The model under review builds one solid part; all positions refer to its coordinate system, in mm. A direction names the side the tool comes from. Round coordinates to 2 decimals unless told otherwise and drop trailing zeros. Order: outer loops, then holes, each group sorted by start corner. A loop starts at its lowest first (then second) coordinate and runs counter-clockwise, first axis right, second up. Notation, with made-up numbers: M 2.25,68.5 L 43.25,68.5 A25 cw 43.25,98.5 Z; hole C 44.5,76.25 d1. An arc over 180 degrees is marked long. Answer as a JSON object with one key per item and string values. Group by question number.
1) For faces 3 (the cylindrical face through (219.16, -261.17, -174.237)), 4 (the flat face through (70, 253, -40)), 5 (the flat face through (281, -266, -164)), 6 (the flat face through (315, 0, 0)), 7 (the flat face through (-4, -250, -1)), list the 3-axis set-ups (+Z, -Z, +X, -X, +Y, -Y) from which the entire face can be reached by the end or side of a thin tool; tool diameter is ignored.
2) Consider section C-C, the plane y = 72.5. Write out the cut boundary in (x, z), then the cut area to 3 significant figures.
3) Consider section A-A, the plane z = -40. Write out the cut boundary in (x, y).
4) Consider section B-B, the plane x = 135.5. Write out the cut boundary in (y, z).
5) To check wall thickness, follow line 1 (X direction, y = 255.5, z = 40); line 2 (Y direction, x = -277, z = -76.5); line 3 (X direction, y = 225, z = -119). State the ranges of each line that lie inside material, in increasing order.
6) Consider section D-D, the plane x = -7. Write out the cut boundary in (y, z).
7) Insertion check: pin 1 Ø5 at (x, z) = (66, -105.5) entering from -Y; pin 2 Ø12 at (y, z) = (-185, -44.5) entering from +X; pin 3 Ø20.5 at (y, z) = (-263.5, -165) entering from -X. Each pin has a flat end and moves straight along its axis. Give the tip position at first contact, or say it passes through.
8) The part is to be moulded in two halves that separate along X. For faces 1 (the flat face through (-1, -251, 175)), 2 (the flat face through (280, -276, -165)), say which applies: +X half, -X half, draft (parallel to the pull), parting line (faces both ways), or undercut.
```python
from build123d import *

# Parameters (mm, degrees)
SKETCH1_W                                  = 600
SKETCH1_H                                  = 500
BOSS_EXTRUDE1_DEPTH                        = 175
SHELL1_T                                   = 10
SKETCH3_W                                  = 620
SKETCH3_H                                  = 360
BOSS_EXTRUDE2_DEPTH                        = 20
SKETCH5_W                                  = 120
SKETCH5_H                                  = 150
CUT_EXTRUDE1_DEPTH                         = 50
BOSS_EXTRUDE3_DEPTH                        = 15
SKETCH9_R                                  = 10
SKETCH9_R_2                                = 8.804977656
SKETCH9_R_3                                = 9.206937975
BOSS_EXTRUDE4_DEPTH                        = 180
BOSS_EXTRUDE8_START                        = -260
BOSS_EXTRUDE8_DEPTH                        = 10
SKETCH147_W                                = 600
SKETCH147_H                                = 15
CUT_EXTRUDE2_DEPTH                         = 10
SKETCH148_R                                = 3.5
BOSS_EXTRUDE10_DEPTH                       = 600
SKETCH149_R                                = 9
CUT_EXTRUDE3_DEPTH                         = 7
MIRROR3_AT_THE_SECOND_PLANE_COPY_1_SKETC_R = 9
MIRROR3_AT_THE_SECOND_PLANE_COPY_1_DEPTH   = 7
SKETCH150_W                                = 60
SKETCH150_H                                = 10
CUT_EXTRUDE4_DEPTH                         = 30
CUT_EXTRUDE10_DEPTH                        = 28
SKETCH155_W                                = 290.489530142
SKETCH155_H                                = 28
CUT_EXTRUDE11_DEPTH                        = 716.53321378
BOSS_EXTRUDE11_DEPTH                       = 488
BOSS_EXTRUDE12_DEPTH                       = 125
BOSS_EXTRUDE12_DEPTH_BACK                  = 445
SKETCH160_W                                = 600
SKETCH160_H                                = 500
CUT_EXTRUDE12_DEPTH                        = 8


with BuildPart() as part:
    # Sketch1 → Boss-Extrude1 (new, symmetric)
    with BuildSketch(Plane.XY):
        Rectangle(SKETCH1_W, SKETCH1_H)
    extrude(amount=BOSS_EXTRUDE1_DEPTH, both=True)

    # Shell1
    shell1_openings = [part.faces().sort_by_distance(p)[0] for p in [
        (0, 0, 175),
    ]]
    offset(amount=SHELL1_T, openings=shell1_openings, kind=Kind.INTERSECTION)

    # Sketch3 → Boss-Extrude2 (add)
    with BuildSketch(Plane.XZ.offset(260)):
        with Locations((0, -5)):
            Rectangle(SKETCH3_W, SKETCH3_H)
    extrude(amount=BOSS_EXTRUDE2_DEPTH)

    # Sketch5 → Cut-Extrude1 (cut)
    with BuildSketch(Plane.XZ.offset(280)):
        with Locations((-170, 100)):
            Rectangle(SKETCH5_W, SKETCH5_H)
        with Locations((170, 100)):
            Rectangle(SKETCH5_W, SKETCH5_H)
        with Locations((-220, -185)):
            Rectangle(SKETCH5_W, SKETCH5_H)
        with Locations((220, -185)):
            Rectangle(SKETCH5_W, SKETCH5_H)
    extrude(amount=-CUT_EXTRUDE1_DEPTH, mode=Mode.SUBTRACT)

    # Sketch8 → Boss-Extrude3 (add, symmetric)
    with BuildSketch(Plane(origin=(0, 0, 0), x_dir=(1, 0, 0), z_dir=(0, 1, 0))):
        Polygon((-310, 10), (-315, 10), (-315, -10), (-310, -10), (-310, -15), (-320, -15), (-320, 15), (-310, 15), align=None)
    boss_extrude3 = extrude(amount=BOSS_EXTRUDE3_DEPTH, both=True)

    # Sketch9 → Boss-Extrude4 (add)
    # profile 1 of 2: a face of its own
    with BuildSketch(Plane.ZY.offset(110)):
        with Locations(Location((155, -265, 0), (0, 0, 180))):
            Circle(SKETCH9_R)
        with Locations((155, -265)):
            Circle(SKETCH9_R_2, mode=Mode.SUBTRACT)
    # profile 2 of 2: a face of its own
    with BuildSketch(Plane.ZY.offset(110)):
        with Locations(Location((-165, -265, 0), (0, 0, 180))):
            Circle(SKETCH9_R)
        with Locations(Location((-165, -265, 0), (0, 0, 180))):
            Circle(SKETCH9_R_3, mode=Mode.SUBTRACT)
    boss_extrude4 = extrude(amount=BOSS_EXTRUDE4_DEPTH)

    # Mirror1: Boss-Extrude3, Boss-Extrude4 across plane
    add(boss_extrude3.mirror(Plane(origin=(0, 0, 0), x_dir=(0, 0, 1), z_dir=(1, 0, 0))))
    add(boss_extrude4.mirror(Plane(origin=(0, 0, 0), x_dir=(0, 0, 1), z_dir=(1, 0, 0))))

    # Sketch17 → Boss-Extrude8 (add, symmetric)
    with BuildSketch(Plane(origin=(0, 260, 0), x_dir=(1, 0, 0), z_dir=(0, 1, 0)).offset(BOSS_EXTRUDE8_START)):
        Polygon((-194.223256177, 185), (-204.223256177, 185), (-204.223256177, 191.540544069), (-159.461030104, 191.540544069), (-159.461030104, 185), (-169.461030104, 185), (-169.461030104, 188.442858537), (-194.223256177, 188.442858537), align=None)
        Polygon((194.223256177, 188.442858537), (194.223256177, 185), (204.223256177, 185), (204.223256177, 191.540544069), (159.461030104, 191.540544069), (159.461030104, 185), (169.461030104, 185), (169.461030104, 188.442858537), align=None)
    extrude(amount=BOSS_EXTRUDE8_DEPTH, both=True)

    # Sketch147 → Cut-Extrude2 (cut)
    with BuildSketch(Plane(origin=(0, 260, 0), x_dir=(1, 0, 0), z_dir=(0, 1, 0))):
        with Locations((0, -167.5)):
            Rectangle(SKETCH147_W, SKETCH147_H)
    extrude(amount=-CUT_EXTRUDE2_DEPTH, mode=Mode.SUBTRACT)

    # Sketch148 → Boss-Extrude10 (add)
    with BuildSketch(Plane(origin=(-300, 0, 0), x_dir=(0, 0, -1), z_dir=(1, 0, 0))):
        with Locations(Location((-168, 255, 0), (0, 0, 180))):
            Circle(SKETCH148_R)
    extrude(amount=BOSS_EXTRUDE10_DEPTH)

    # Sketch149 → Cut-Extrude3 (cut)
    with BuildSketch(Plane(origin=(0, 260, 0), x_dir=(1, 0, 0), z_dir=(0, 1, 0))):
        with Locations(Location((-70, 40, 0), (0, 0, 270))):
            Circle(SKETCH149_R)
    cut_extrude3 = extrude(amount=-CUT_EXTRUDE3_DEPTH, mode=Mode.SUBTRACT)

    # Mirror3: Cut-Extrude3 across plane
    add(cut_extrude3.mirror(Plane.XY), mode=Mode.SUBTRACT)

    # Mirror3 at the second plane: Cut-Extrude3 across plane
    add(cut_extrude3.mirror(Plane(origin=(0, 0, 0), x_dir=(0, 0, 1), z_dir=(1, 0, 0))), mode=Mode.SUBTRACT)

    # Mirror3 at the second plane copy 1 sketc → Mirror3 at the second plane copy 1 (cut)
    with BuildSketch(Plane(origin=(0, 260, 0), x_dir=(-1, 0, 0), z_dir=(0, 1, 0))):
        with Locations(Location((-70, 40, 0), (0, 0, 270))):
            Circle(MIRROR3_AT_THE_SECOND_PLANE_COPY_1_SKETC_R)
    extrude(amount=-MIRROR3_AT_THE_SECOND_PLANE_COPY_1_DEPTH, mode=Mode.SUBTRACT)

    # Sketch150 → Cut-Extrude4 (cut)
    with BuildSketch(Plane.XY.offset(175)):
        with Locations((0, -259)):
            Rectangle(SKETCH150_W, SKETCH150_H)
    extrude(amount=-CUT_EXTRUDE4_DEPTH, mode=Mode.SUBTRACT)

    # Sketch154 → Cut-Extrude10 (cut)
    with BuildSketch(Plane.XZ.offset(280)):
        Polygon((309, -184), (309, 174), (231, 174), (231, 24), (109, 24), (109, 174), (-109, 174), (-109, 24), (-231, 24), (-231, 174), (-309, 174), (-309, -184), (-281, -184), (-281, -109), (-159, -109), (-159, -184), (159, -184), (159, -109), (281, -109), (281, -184), align=None)
    extrude(amount=-CUT_EXTRUDE10_DEPTH, mode=Mode.SUBTRACT)

    # Sketch155 → Cut-Extrude11 (cut, through all)
    with BuildSketch(Plane.ZY.offset(310)):
        with Locations((0, -266)):
            Rectangle(SKETCH155_W, SKETCH155_H)
    extrude(amount=-CUT_EXTRUDE11_DEPTH, mode=Mode.SUBTRACT)

    # Sketch157 → Boss-Extrude11 (add)
    with BuildSketch(Plane(origin=(-230, 0, 0), x_dir=(0, 0, -1), z_dir=(1, 0, 0))):
        Polygon((-145.244765071, -252), (-175, -252), (-175, -250), (-25, -250), (-25, -252), align=None)
    extrude(amount=BOSS_EXTRUDE11_DEPTH)

    # Sketch159 → Boss-Extrude12 (add, two sides: drawn at the far end of the back side and taken through both)
    with BuildSketch(Plane(origin=(160, 0, 0), x_dir=(0, 0, -1), z_dir=(1, 0, 0)).offset(-BOSS_EXTRUDE12_DEPTH_BACK)):
        Polygon((145.244765071, -252), (185, -252), (185, -230), (175, -230), (175, -250), (110, -250), (110, -252), align=None)
    extrude(amount=BOSS_EXTRUDE12_DEPTH + BOSS_EXTRUDE12_DEPTH_BACK)

    # Sketch160 → Cut-Extrude12 (cut)
    with BuildSketch(Plane.XY.offset(-175)):
        Rectangle(SKETCH160_W, SKETCH160_H)
    extrude(amount=-CUT_EXTRUDE12_DEPTH, mode=Mode.SUBTRACT)


solid = part.part
```
Results list:
{
 "1": {"face 3": "none", "face 4": "+Y", "face 5": "-Y", "face 6": "+Y, -Y", "face 7": "+Z"},
 "2": {"outline": "M -310,-185 L 310,-185 L 310,175 L 300,175 L 300,-183 L -300,-183 L -300,175 L -310,175 Z", "area": "8,400 mm^2"},
 "3": {"outline": "M -310,-252 L 310,-252 L 310,260 L 79,260 L 79,253 L 61,253 L 61,260 L -61,260 L -61,253 L -79,253 L -79,260 L -310,260 Z; hole M -300,-250 L 300,-250 L 300,250 L -300,250 Z"},
 "4": {"outline": "M -280,-185 L 260,-185 L 260,160 L 250,160 L 250,-183 L -250,-183 L -250,175 L -252,175 L -252,-184 L -280,-184 Z; M -267.2,145.24 L -262.8,145.24 A10 ccw long Z; C 255,168 d7; hole C -265,155 d17.61"},
 "5": {"line 1": "-310 to -79, -61 to 61, 79 to 310", "line 2": "-252 to -250, 250 to 260", "line 3": "-310 to -300, 300 to 310"},
 "6": {"outline": "M -280,-185 L 260,-185 L 260,160 L 250,160 L 250,-183 L -250,-183 L -250,175 L -254,175 L -254,174 L -252,174 L -252,-184 L -280,-184 Z; M -280,174 L -264,174 L -264,175 L -280,175 Z; C 255,168 d7"},
 "7": {"pin 1": "y = -252", "pin 2": "x = 310", "pin 3": "x = -310"},
 "8": {"face 1": "draft", "face 2": "undercut"}
}
